Autodesk Inventor part; units mm, degrees
ref_plane "YZ Plane" through (0, 0, 0) normal (1, 0, 0) x (0, 1, 0)
ref_plane "XZ Plane" through (0, 0, 0) normal (0, 1, 0) x (-1, 0, 0)
ref_plane "XY Plane" through (0, 0, 0) normal (0, 0, 1) x (1, 0, 0)
sketch "Sketch1" plane through (0, 0, 0) normal (0, 1, 0) x (-1, 0, 0)
  circle A0 centre (0, 0) radius 12 construction
  line L0 (0, 0) -> (0, -50) construction
  line L1 (20, -50) -> (34, -50) construction
  line L2 (34, -50) -> (34, -16) construction
  line L3 (34, -16) -> (20, -16) construction
  line L4 (20, -16) -> (20, -50) construction
  arc A1 (-2.3199, 5.5334) -> (0, -6) centre (0, 0) ccw
  arc A2 (17.5, -16.3175) -> (0, -6) centre (0, -26) ccw
  arc A3 (35.3201, -7.2377) -> (-2.3199, 5.5334) centre (9.2795, -22.1335) ccw
  circle A4 centre (0, 0) radius 2
  line L5 (17.5, -16.3175) -> (35.3201, -7.2377)
  point P0 (16, -42)
  point P1 (39, -42)
  point P2 (16, -14)
  dimension "d0" = 50
  dimension "d1" = 24
  dimension "d16" = 16
  dimension "d17" = 34
  dimension "d18" = 23
  dimension "d23" = 20
  dimension "d26" = 12
  dimension "d32" = 20
  dimension "d33" = 4
  dimension "d34" = 30
  dimension "d35" = 2.5
  dimension "d36" = 14
  dimension "d37" = 27
  dimension "d38" = 20
extrude "Extrusion1" add sketch "Sketch1" along normal blind 2
properties part number "flange_connector"
Design review of the part built by this model. Coordinates are the model's own, in mm. Give positions to 0.01 mm unless a question says otherwise; leave off trailing zeros. Order: outer loops, then holes, each group sorted by start corner. A loop starts at its lowest first (then second) coordinate and runs counter-clockwise, first axis right, second up. Notation, with made-up numbers: (43.25, 15) -> (90.25, 15) arc R16 cw to (90.25, 44) -> close; hole circle Ø8 at (32.25, 19). An arc over 180 degrees is marked (long way). Write item = value, one per line. Start each with the question number.
(1) We need section B-B on x = 0.5. Write out the cut boundary in (y, z), plus the area to 3 significant figures.
(2) We need section C-C on y = 0.5. Write out the cut boundary in (x, z).
(3) We need section A-A on z = 0.75. Write out the cut boundary in (x, y).
(4) Mouldability with a two-part tool opening along X and no side actions: class faces 1 (the face through (-26.29, 0.99, -11.84)), 2 (the face through (-14, 0, -1)), 3 (the face through (0, 1, 2)) as +X half, -X half, draft (parallel to the pull), parting line (faces both ways), or undercut.
(5) We need section D-D on z = -4.5. Write out the cut boundary in (x, y), plus the area to 3 significant figures.
(6) To check wall thickness, follow line 1 along X through (y, z) = (1.5, 1); line 2 along Z through (x, y) = (0, 0.7); line 3 along Z through (x, y) = (1.5, 1.4). State the ranges of each line that lie inside material, in increasing order.
Numbers:
q1.outline = (0, -5.98) -> (2, -5.98) -> (2, -1.94) -> (0, -1.94) -> close; (0, 1.94) -> (2, 1.94) -> (2, 6.23) -> (0, 6.23) -> close
q1.area = 16.7 mm^2
q2.outline = (-35.32, -7.24) -> (-17.5, -16.32) arc R20 cw to (0, -6) arc R6 ccw to (2.32, 5.53) arc R30 ccw to start; hole circle Ø4 at (0, 0)
q3.outline = (-28.68, 0) -> (-1.85, 0) -> (-1.85, 2) -> (-28.68, 2) -> close; (1.85, 0) -> (5.95, 0) -> (5.95, 2) -> (1.85, 2) -> close
q4.face_1 = -X half
q4.face_2 = draft
q4.face_3 = undercut
q5.outline = (-33.55, 0) -> (3.97, 0) -> (3.97, 2) -> (-33.55, 2) -> close
q5.area = 75.0 mm^2
q6.line_1 = -28.38 to -1.73, 1.73 to 5.92
q6.line_2 = -6 to -2, 2 to 6.4
q6.line_3 = -5.81 to -1.32, 1.32 to 5.86
